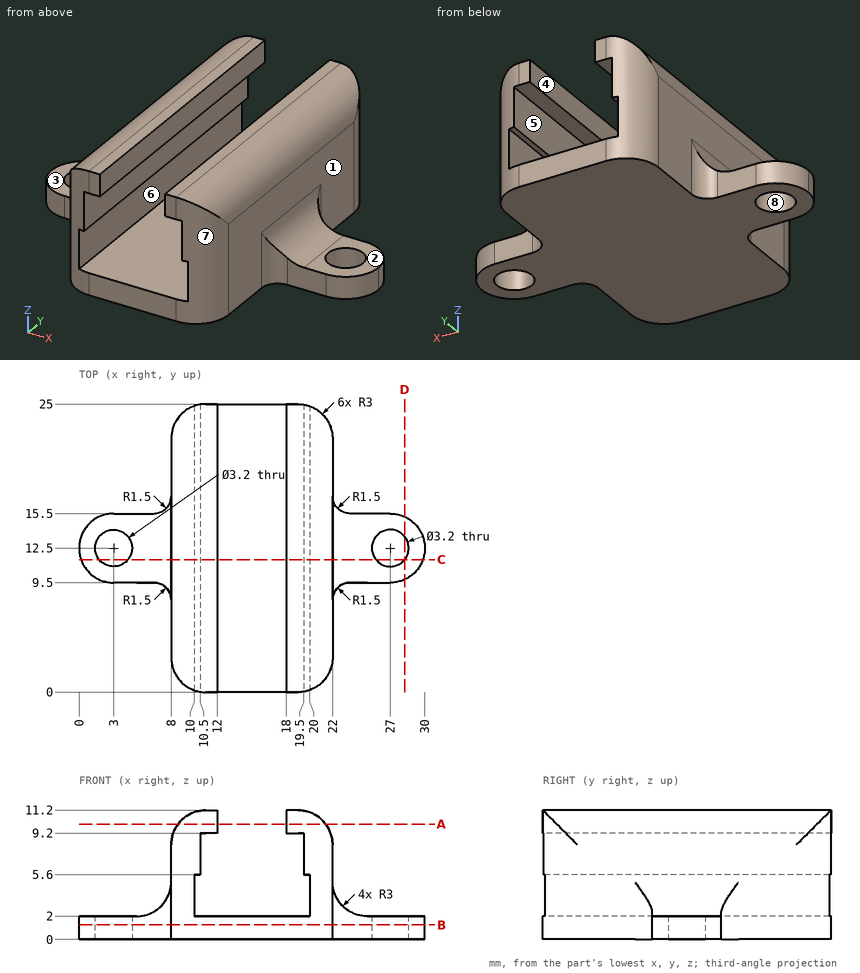
Check sheet for the drawn part. Datum: minimum x, y, z corner. Units: mm. A direction names the side the tool comes from. Coordinates: 2 decimals unless noted, no trailing zeros. Loops run counter-clockwise (first coordinate to the right, second up) from the corner with the lowest first, then second, coordinate; pieces in that order, holes last. Notation, with made-up numbers: (56.5, 39.25) -> (66.5, 39.25) arc R23 cw to (66.5, 53.25) -> close; hole circle Ø3 at (14.25, -33.5). An arc over 180 degrees is marked (long way). Answer as a JSON object with one key per item and string values. Group by question number.
Item 1: Sectioned sample at A-A on z = 10. Record the boundary of the cut face in (x, y).
Item 2: Sectioned sample at B-B on z = 1.25. Record the boundary of the cut face in (x, y), plus the area to 3 significant figures.
Item 3: Mould release check, pull along Y, two halves, no side actions. Record for the marked faces 6, 7 and 8: +Y half, -Y half, draft (parallel to the pull), parting line (faces both ways), or undercut.
Item 4: Sectioned sample at D-D on x = 28.25. Record the boundary of the cut face in (y, z), plus the area to 3 significant figures.
Item 5: Depth check by flat-ended pin: pin 1 (4 mm diameter, centred on y = 9.5, z = 7, fed in from -X); pin 2 (1.5 mm diameter, centred on x = 16, y = 10, fed in from +Z); pin 3 (1.2 mm diameter, centred on x = 4, z = 1.5, fed in from +Y). Enter the tip coordinate at first touch or a pass-through.
Item 6: Scan lines: probe 1 along Y at (x, z) = (27, 1.5); probe 2 along Z at (x, y) = (18.75, 6); probe 3 along Z at (x, y) = (10.25, 17.75). Record each from-to range of solid material in increasing order.
Item 7: Tool access check on the marked faces 1, 2, 3, 4 and 5. Record the directions out of +Z, -Z, +X, -X, +Y, -Y that give a thin tool (end or side, any length) a straight path to the whole face; none if there is none.
Item 8: Sectioned sample at C-C on y = 11.5. State how many separate pieces and enclosed holes the cut face has, plus the area to 3 significant figures.
Evaluation:
{
 "1": {"outline": "(8.6, 1.2) arc R3 ccw to (11, 0) -> (12, 0) -> (12, 25) -> (11, 25) arc R3 ccw to (8.6, 23.8) -> close; (18, 0) -> (19, 0) arc R3 ccw to (21.4, 1.2) -> (21.4, 23.8) arc R3 ccw to (19, 25) -> (18, 25) -> close"},
 "2": {"outline": "(3, 9.5) -> (6.5, 9.5) arc R1.5 cw to (8, 8) -> (8, 3) arc R3 ccw to (11, 0) -> (19, 0) arc R3 ccw to (22, 3) -> (22, 8) arc R1.5 cw to (23.5, 9.5) -> (27, 9.5) arc R3 ccw to (27, 15.5) -> (23.5, 15.5) arc R1.5 cw to (22, 17) -> (22, 22) arc R3 ccw to (19, 25) -> (11, 25) arc R3 ccw to (8, 22) -> (8, 17) arc R1.5 cw to (6.5, 15.5) -> (3, 15.5) arc R3 ccw to start; hole circle Ø3.2 at (3, 12.5); hole circle Ø3.2 at (27, 12.5)", "area": "416 mm²"},
 "3": {"face 6": "draft", "face 7": "-Y half", "face 8": "undercut"},
 "4": {"outline": "(9.77, 0) -> (11.5, 0) -> (11.5, 2) -> (9.77, 2) -> close; (13.5, 0) -> (15.23, 0) -> (15.23, 2) -> (13.5, 2) -> close", "area": "6.91 mm²"},
 "5": {"pin 1": "stops at x = 8", "pin 2": "stops at z = 2", "pin 3": "stops at y = 15.5"},
 "6": {"probe 1": "y = 9.5 to 10.9, 14.1 to 15.5", "probe 2": "z = 0 to 2, 9.2 to 11.2", "probe 3": "z = 0 to 2, 5.6 to 11.1"},
 "7": {"face 1": "+Z, +X", "face 2": "+Z, +X, +Y, -Y", "face 3": "+Z, -X, +Y, -Y", "face 4": "+Z, +Y, -Y", "face 5": "+Y, -Y"},
 "8": {"separate pieces": "3", "enclosed holes": "0", "area": "97.7 mm²"}
}
